Drawing for the job (mm, zero at the part's lowest x, y, z). A direction names the side the tool comes from. Round coordinates to 2 decimals unless told otherwise and drop trailing zeros. Write each loop counter-clockwise with the first axis right and the second up, starting at its lowest first coordinate (ties: lowest second). Pieces come first, ordered by that corner, then holes. Notation, with made-up numbers: M 69,54.5 L 107,54.5 A17 ccw 107,60.5 Z; hole C 13.25,41.25 d10. An arc over 180 degrees is marked long. Use a Markdown table: item, result.
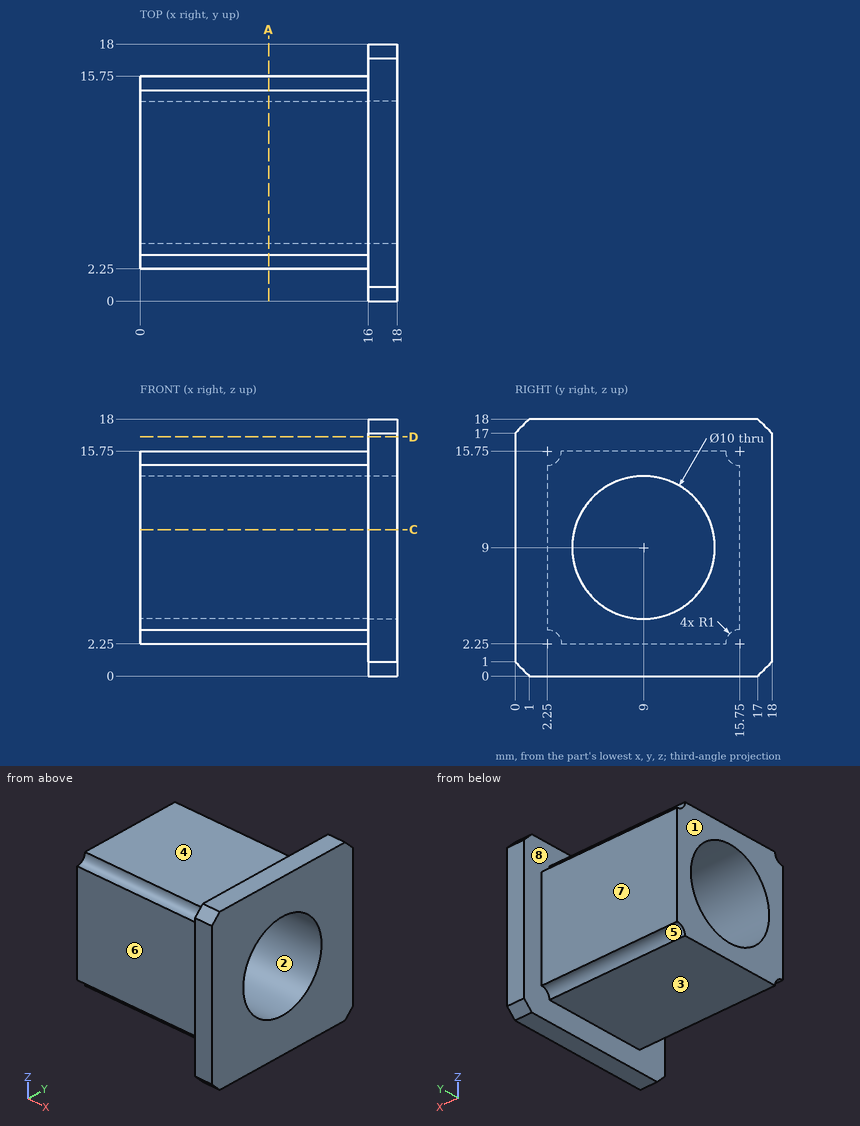
Q1. Which spindle directions (+Z, -Z, +X, -X, +Y, -Y) get a long thin tool onto all of the face, cutting with end or side? Do the marked faces 5, 6, 7 and 8. Say none if no direction does.
Response values:
| item | result |
|---|---|
| face 5 | -Z, -X, +Y |
| face 6 | +Z, -Z, -X, -Y |
| face 7 | +Z, -Z, -X, +Y |
| face 8 | -X |
Q2. Cut at A-A on x = 9. Give the cut face in (y, z), and give its area (3 significant figures).
Response values:
| item | result |
|---|---|
| outline | M 2.25,3.25 A1 cw 3.25,2.25 L 14.75,2.25 A1 cw 15.75,3.25 L 15.75,14.75 A1 cw 14.75,15.75 L 3.25,15.75 A1 cw 2.25,14.75 Z; hole C 9,9 d10 |
| area | 101 mm2 |
Q3. Drop flat-ended pins along their axis: P1, Ø10, axis at x = 2.5, z = 14, coming from the +Y side; P2, Ø9, axis at y = 9, z = 9, coming from the +X side (3 decimals); P3, Ø3, axis at x = 10, y = 10, coming from the -Z side; P4, Ø2, axis at x = 13.5, y = 16, coming from the -Z side. Give the stop position or say it passes through.
Response values:
| item | result |
|---|---|
| P1 | stops at y = 15.75 |
| P2 | passes through |
| P3 | stops at z = 2.25 |
| P4 | stops at z = 2.91 |
Q4. Drill centre lines: L1, parallel to Y at x = 8.5, z = 9; L2, parallel to X at y = 16, z = 12.75. Where is each one in solid material? Low to high.
Response values:
| item | result |
|---|---|
| L1 | y = 2.25 to 4, 14 to 15.75 |
| L2 | x = 16 to 18 |
Q5. Cut at C-C on z = 10.25. Give the cut face in (x, y).
Response values:
| item | result |
|---|---|
| outline | M 0,2.25 L 16,2.25 L 16,0 L 18,0 L 18,4.16 L 0,4.16 Z; M 0,13.84 L 18,13.84 L 18,18 L 16,18 L 16,15.75 L 0,15.75 Z |
Q6. Cut at D-D on z = 16.75. Give the cut face in (x, y), and give its area (3 significant figures).
Response values:
| item | result |
|---|---|
| outline | M 16,0 L 18,0 L 18,18 L 16,18 Z |
| area | 36.0 mm2 |
Q7. Two-plate mould, pull along Z, no slides. Class the marked faces 1, 2, 3 and 4: +Z half, -Z half, draft (parallel to the pull), parting line (faces both ways), or undercut.
Response values:
| item | result |
|---|---|
| face 1 | draft |
| face 2 | undercut |
| face 3 | -Z half |
| face 4 | +Z half |
